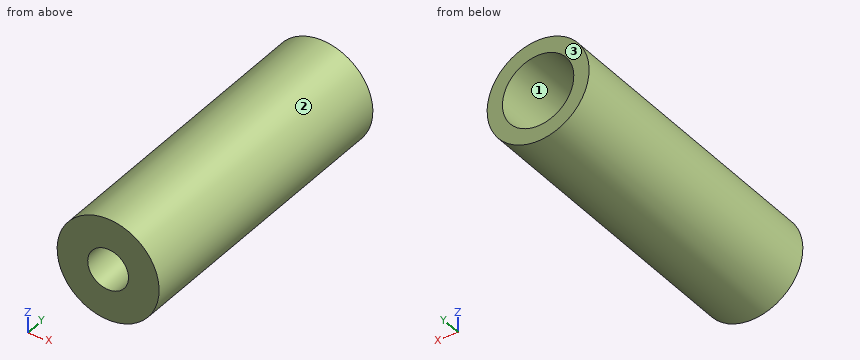
from build123d import *

# Parameters (mm, degrees)
SKETCH1_R           = 5
BOSS_EXTRUDE1_DEPTH = 30
CUT_EXTRUDE1_REACH  = 32.822
SKETCH2_R           = 2
SKETCH3_R           = 3.5
CUT_EXTRUDE2_DEPTH  = 25


with BuildPart() as part:
    # Sketch1 → Boss-Extrude1 (new body)
    with BuildSketch(Plane(origin=(0, 0, 0), x_dir=(1, 0, 0), z_dir=(0, 1, 0))):
        with Locations(Location((0, 0, 0), (0, 0, 270))):
            Circle(SKETCH1_R)
    extrude(amount=BOSS_EXTRUDE1_DEPTH)

    # Sketch2 → Cut-Extrude1 (cut, up to next)
    with BuildSketch(Plane(origin=(0, 30, 0), x_dir=(1, 0, 0), z_dir=(0, 1, 0)), mode=Mode.PRIVATE) as cut_extrude1_sk1:
        with Locations(Location((0, 0, 0), (0, 0, 270))):
            Circle(SKETCH2_R)
    cut_extrude1_tool1 = extrude(cut_extrude1_sk1.sketch, amount=-CUT_EXTRUDE1_REACH, mode=Mode.PRIVATE) & part.part
    add(cut_extrude1_tool1.solids().sort_by_distance((0, 30, 0))[0], mode=Mode.SUBTRACT)

    # Sketch3 → Cut-Extrude2 (cut)
    with BuildSketch(Plane(origin=(0, 30, 0), x_dir=(1, 0, 0), z_dir=(0, 1, 0))):
        with Locations(Location((0, 0, 0), (0, 0, 270))):
            Circle(SKETCH3_R)
    extrude(amount=-CUT_EXTRUDE2_DEPTH, mode=Mode.SUBTRACT)


solid = part.part
Verification items for the finished model (mm, model axes). Face numbers are marked on the shaded views. Round coordinates to 2 decimals unless told otherwise and drop trailing zeros. Loops run counter-clockwise (first coordinate to the right, second up) from the corner with the lowest first, then second, coordinate; pieces in that order, holes last. Notation, with made-up numbers: (62, 18) - (82, 18) arc R17 cw to (82, 34) - close; hole circle Ø9 at (41, 19.5). An arc over 180 degrees is marked (long way). Use a Markdown table: item, result. Add a question column.
1. Gauge pin test, flat ends, axial feed: pin 1 (2 mm diameter, centred on x = -1.5, z = -1.5, fed in from +Y); pin 2 (3 mm diameter, centred on x = -2.5, y = 11.5, fed in from -Z); pin 3 (3 mm diameter, centred on x = -2.5, y = 5.5, fed in from +Z). Record the tip position at first contact, or that the pin passes through.
2. Thickness scan on probe 1 along X at (y, z) = (3.2, 0); probe 2 along X at (y, z) = (15.75, -1.5); probe 3 along Y at (x, z) = (-1, -2). Record the ranges inside material, lowest first. Write a range as [from, to].
3. Section check C-C, the plane x = -0.5. Record the boundary of the cut face in (y, z), plus the area to 3 significant figures.
4. Release check for a two-part mould opening along Z. For the marked faces 1, 2 and 3 record: released by +Z, released by -Z, zero draft, split by the parting line, or undercut.
5. Section check A-A, the plane z = 0. Record the boundary of the cut face in (x, y), plus the area to 3 significant figures.
6. Section check D-D, the plane x = 4. Record the boundary of the cut face in (y, z).
7. Section check B-B, the plane y = 26. Record the boundary of the cut face in (x, z), plus the area to 3 significant figures.
Checks:
| question | item | result |
|---|---|---|
| 1 | pin 1 | stops at y = 5 |
| 1 | pin 2 | stops at z = -4.9 |
| 1 | pin 3 | stops at z = 4.9 |
| 2 | probe 1 | x = [-5, -2], [2, 5] |
| 2 | probe 2 | x = [-4.77, -3.16], [3.16, 4.77] |
| 2 | probe 3 | y = [0, 5] |
| 3 | outline | (0, -4.97) - (30, -4.97) - (30, -3.46) - (5, -3.46) - (5, -1.94) - (0, -1.94) - close; (0, 1.94) - (5, 1.94) - (5, 3.46) - (30, 3.46) - (30, 4.97) - (0, 4.97) - close |
| 3 | area | 106 mm^2 |
| 4 | face 1 | undercut |
| 4 | face 2 | split by the parting line |
| 4 | face 3 | zero draft |
| 5 | outline | (-5, 0) - (-2, 0) - (-2, 5) - (-3.5, 5) - (-3.5, 30) - (-5, 30) - close; (2, 0) - (5, 0) - (5, 30) - (3.5, 30) - (3.5, 5) - (2, 5) - close |
| 5 | area | 105 mm^2 |
| 6 | outline | (0, -3) - (30, -3) - (30, 3) - (0, 3) - close |
| 7 | outline | circle Ø10 at (0, 0); hole circle Ø7 at (0, 0) |
| 7 | area | 40.1 mm^2 |
